Drawing for the job (mm, zero at the part's lowest x, y, z). A direction names the side the tool comes from. Round coordinates to 2 decimals unless told otherwise and drop trailing zeros. Loops run counter-clockwise (first coordinate to the right, second up) from the corner with the lowest first, then second, coordinate; pieces in that order, holes last. Notation, with made-up numbers: (35, 43.25) -> (89, 43.25) arc R16 ccw to (89, 47.25) -> close; hole circle Ø4 at (45.25, 8). An arc over 180 degrees is marked (long way). Put each result on its own line as item: value. Start each with the question number.
Item 1: Flat gauge pins, fed straight in: pin 1 Ø2 at (x, y) = (2.5, 3) entering from +Z; pin 2 Ø1 at (x, z) = (1.5, 5.5) entering from +Y; pin 3 Ø1.5 at (y, z) = (1, 4) entering from +X; pin 4 Ø3 at (y, z) = (2, 4) entering from +X. Where does each tip first touch, or does it go through?
Item 2: Tool access for the marked faces 1 and 2: list every direction of +Z, -Z, +X, -X, +Y, -Y with a clear straight run to the whole face (end or side of a thin tool).
Item 3: Cut at B-B, the plane z = 3.8. List the corners of the cut face in (x, y), plus the area to 3 significant figures.
Item 4: Drill centre lines: probe 1 along Z at (x, y) = (6.5, 2.25); probe 2 along Y at (x, z) = (4, 5.6) (3 decimals); probe 3 along Y at (x, z) = (7.5, 2.15). Where is each one in solid material? Low to high. Write a range as [from, to].
Item 5: Cut at A-A, the plane x = 4. List the corners of the cut face in (y, z) (3 decimals), plus the area to 3 significant figures.
Item 6: Cut at C-C, the plane z = 5.1. List the corners of the cut face in (x, y) (3 decimals).
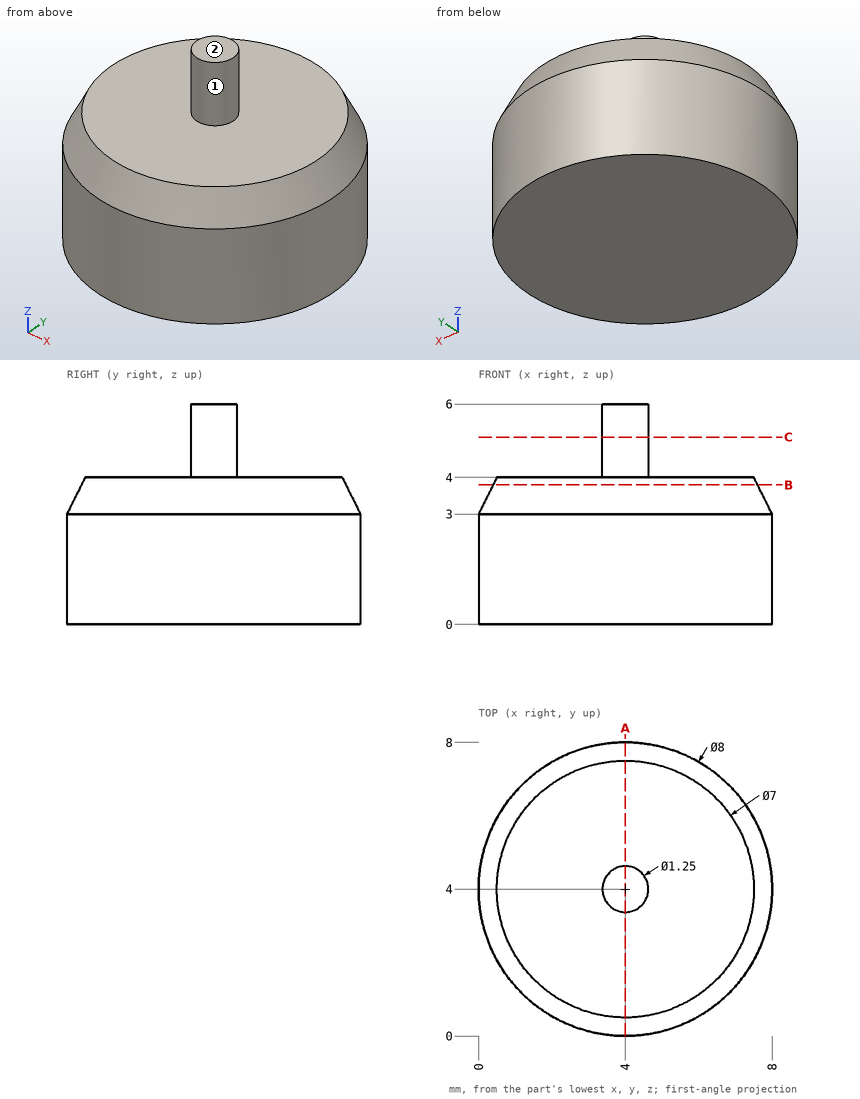
Reply:
1. pin 1: stops at z = 4
1. pin 2: passes through
1. pin 3: stops at x = 6.85
1. pin 4: stops at x = 7.9
2. face 1: +Z
2. face 2: +Z, +X, -X, +Y, -Y
3. outline: circle Ø7.2 at (4, 4)
3. area: 40.7 mm^2
4. probe 1: z = [0, 4]
4. probe 2: y = [3.375, 4.625]
4. probe 3: y = [2.06, 5.94]
5. outline: (0, 0) -> (8, 0) -> (8, 3) -> (7.5, 4) -> (4.625, 4) -> (4.625, 6) -> (3.375, 6) -> (3.375, 4) -> (0.5, 4) -> (0, 3) -> close
5. area: 34.0 mm^2
6. outline: circle Ø1.25 at (4, 4)
